Read the model definition and answer for the solid it produces. Units are mm, in the model's axes. A direction names the side the tool comes from. Give positions to 0.01 mm unless a question says otherwise; leave off trailing zeros. Order: outer loops, then holes, each group sorted by start corner. A loop starts at its lowest first (then second) coordinate and runs counter-clockwise, first axis right, second up. Notation, with made-up numbers: (21, 87) - (58, 87) arc R13 ccw to (58, 95) - close; hole circle Ø4 at (58.5, -40). An arc over 180 degrees is marked (long way). Use a Markdown table: item, result. Add a question column.
1. Which of the six approach directions +Z, -Z, +X, -X, +Y, -Y give full straight-line access (tool end or side, diameter ignored) to faces 1 (the flat face through (10, 23, -148)), 2 (the cylindrical face through (240.07, 23.612, -206.105))?
2. Consider L1, parallel to X at y = 21, z = -42; L2, parallel to Y at x = 7.75, z = -220; L3, parallel to Z at x = 239.5, y = 23. Determine where each line is inside the solid, lowest interval first.
3. Flat-ended cylindrical pins translate along their axes: P1, Ø22.5, axis at y = 23, z = -220, coming from the -X side; P2, Ø3, axis at x = 106.5, z = -238.5, coming from the +Y side. Find the tip coordinate at first contact, or state that the pin passes through.
4. A cutting plane is placed at A-A on y = 23. Determine the outline of the cut face in (x, z), and give its area (3 significant figures).
5. A cutting plane is placed at C-C on x = 114. Determine the outline of the cut face in (y, z), and give its area (3 significant figures).
6. For a pull along Y with two mould halves and no side action, classify faces 3 (the cylindrical face through (5.07, 23.612, -206.105)), 4 (the flat face through (124, 19, 0)), 5 (the flat face through (121, 8, -152)) as released by +Y, released by -Y, zero draft, split by the parting line, or undercut.
7. A cutting plane is placed at D-D on z = -68. Determine the outline of the cut face in (x, y).
8. A cutting plane is placed at B-B on z = -220. Determine the outline of the cut face in (x, y).
Autodesk Inventor part; units mm, degrees
ref_plane "YZ Plane" through (0, 0, 0) normal (1, 0, 0) x (0, 1, 0)
ref_plane "XZ Plane" through (0, 0, 0) normal (0, 1, 0) x (-1, 0, 0)
ref_plane "XY Plane" through (0, 0, 0) normal (0, 0, 1) x (1, 0, 0)
sketch "Sketch1" plane through (0, 0, 0) normal (0, 1, 0) x (-1, 0, 0)
  line L0 (0, 0) -> (0, -250)
  line L1 (-200, 0) -> (0, 0)
  line L2 (0, -250) -> (0, -300)
  line L3 (0, -300) -> (-200, -300)
  line L4 (-200, -300) -> (-230, -300)
  line L5 (-230, 0) -> (-200, 0)
  line L6 (-230, -300) -> (-245, -300)
  line L7 (-245, -300) -> (-245, 0)
  line L8 (-245, 0) -> (-230, 0)
  dimension "d0" = 250
  dimension "d4" = 50
  dimension "d12" = 30
  dimension "d24" = 15
extrude "Extrusion1" add sketch "Sketch1" along normal blind 38
sketch "Sketch2" plane through (0, 38, 0) normal (0, 1, 0) x (1, 0, 0)
  line L0 (0, 300) -> (0, 0)
  line L1 (0, 0) -> (245, 0)
  line L2 (10, 10) -> (10, 290)
  line L3 (245, 300) -> (0, 300)
  line L4 (245, 0) -> (245, 300)
  line L5 (245, 290) -> (235, 290)
  line L6 (235, 290) -> (235, 10)
  line L7 (235, 290) -> (10, 290)
  line L8 (0, 300) -> (0, 0)
  line L9 (235, 10) -> (10, 10)
  dimension "d25" = 10
extrude "Extrusion2" cut sketch "Sketch2" against normal blind 30 contours L6 L9 L2 L7
sketch "Sketch5" plane through (0, 0, 0) normal (0, -1, 0) x (1, 0, 0)
  point P0 (0, 0)
sketch "Sketch6" plane through (0, 8, 0) normal (0, 1, 0) x (1, 0, 0)
  point P0 (0, 0)
sketch "Sketch7" plane through (0, 8, 0) normal (0, 1, 0) x (1, 0, 0)
  line L0 (10, 290) -> (235, 290)
  line L1 (235, 10) -> (10, 10)
  line L2 (235, 290) -> (10, 10)
  line L3 (10, 10) -> (10, 290)
  line L4 (235, 10) -> (10, 290)
  point P0 (0, 0)
sketch "Sketch8" plane through (245, 0, 0) normal (1, 0, 0) x (0, 0, -1)
  line L0 (0, 38) -> (300, 38)
  line L1 (0, 0) -> (300, 0)
  line L2 (0, 0) -> (0, 38)
  line L3 (150, 38) -> (150, 8)
  line L4 (290, 8) -> (10, 8)
  line L5 (150, 8) -> (290, 8)
  line L6 (290, 38) -> (290, 8)
  line L7 (290, 8) -> (290, 38)
  line L8 (290, 38) -> (150, 38)
  line L9 (290, 38) -> (10, 38)
  line L10 (150, 8) -> (290, 38)
  line L11 (290, 38) -> (150, 38)
  line L12 (290, 8) -> (150, 38)
  circle A0 centre (220, 23) radius 13.9087
extrude "Extrusion4" cut sketch "Sketch8" against normal blind 250 contours A0 L10 L12 | L12 L10 A0 | A0 L12 L10 | L10 L12 A0
equation "\"BendRadius\" = Thickness"
equation "\"BendReliefWidth\" = Thickness"
equation "\"BendReliefDepth\" = 0.5 * Thickness"
equation "\"CornerReliefSize\" = 4 * Thickness"
equation "\"MinimumRemnant\" = 2 * Thickness"
equation "\"TransitionRadius\" = BendRadius"
equation "\"JacobiRadiusSize\" = BendRadius"
equation "\"GapSize\" = Thickness"
properties part number "Case_3d_model_3DPrint"
Output values:
| question | item | result |
|---|---|---|
| 1 | face 1 | +Y |
| 1 | face 2 | +X, -X |
| 2 | L1 | 0 to 10, 235 to 245 |
| 2 | L2 | 0 to 9.09, 36.91 to 38 |
| 2 | L3 | -300 to -233.91, -206.09 to 0 |
| 3 | P1 | through |
| 3 | P2 | y = 8 |
| 4 | outline | (0, -300) - (245, -300) - (245, -233.91) - (235, -233.91) - (235, -290) - (10, -290) - (10, -233.91) - (0, -233.91) - close; (0, -206.09) - (10, -206.09) - (10, -10) - (235, -10) - (235, -206.09) - (245, -206.09) - (245, 0) - (0, 0) - close |
| 4 | area | 9,940 mm² |
| 5 | outline | (0, -300) - (38, -300) - (38, -290) - (8, -290) - (8, -10) - (38, -10) - (38, 0) - (0, 0) - close |
| 5 | area | 3,000 mm² |
| 6 | face 3 | undercut |
| 6 | face 4 | zero draft |
| 6 | face 5 | released by +Y |
| 7 | outline | (0, 0) - (245, 0) - (245, 38) - (235, 38) - (235, 8) - (10, 8) - (10, 38) - (0, 38) - close |
| 8 | outline | (0, 0) - (245, 0) - (245, 9.09) - (235, 9.09) - (235, 8) - (10, 8) - (10, 9.09) - (0, 9.09) - close; (0, 36.91) - (10, 36.91) - (10, 38) - (0, 38) - close; (235, 36.91) - (245, 36.91) - (245, 38) - (235, 38) - close |
